Part model, mm, in its own coordinate system. Coordinates: 2 decimals unless noted, no trailing zeros. Write each loop counter-clockwise with the first axis right and the second up, starting at its lowest first coordinate (ties: lowest second). Pieces come first, ordered by that corner, then holes. Notation, with made-up numbers: (41, 80.5) -> (63, 80.5) arc R29 cw to (63, 118.5) -> close; hole circle Ø6 at (-13.75, 14.5). An arc over 180 degrees is marked (long way). Write item = value, one per line. Start each with the question number.
Q1. Band-saw the part on A-A, the plane y = 0. List the corners of the cut face in (x, z), plus the area to 3 significant figures.
Q2. Pull direction X, two halves, no side cores. Call faces 1 (the flat face through (-2, 0, 0.5)), 2 (the cylindrical face through (-1.216, 1.115, 0.303)): released by +X, released by -X, zero draft, split by the parting line, or undercut.
Q3. Pin check, flat tip, straight feed: P1, Ø1, axis at x = 0.5, y = -1, coming from the +Z side. Stop position of the tip, or through.
Q4. Probe line 1 (Y direction, x = 0, z = 0.2); line 2 (Y direction, x = 0.75, z = 0.3); line 3 (Y direction, x = 4, z = 0.15). List the from-to ranges inside material, lowest first.
from build123d import *

# Parameters (mm, degrees)
F0_R     = 7.5
F1_DEPTH = 0.5
F2_R     = 0.15
F3_R     = 1.65
F4_DEPTH = 0.4


# Not quite as in the source:
# - a feature names something its author has since deleted; it is built from what else it names


with BuildPart() as f1:
    # F0 (on Top) → F1 (new body)
    with BuildSketch(Plane.XY):
        Circle(F0_R)
    extrude(amount=F1_DEPTH)

    # F2
    f2_edges = [f1.edges().sort_by_distance(p)[0] for p in [
        (-7.5, 0, 0.5),
        (-7.5, 0, 0),
    ]]
    fillet(f2_edges, radius=F2_R)

    # F3 (on face) → F4 (cut)
    with BuildSketch(Plane.XY.offset(0.5)):
        Circle(F3_R)
    extrude(amount=-F4_DEPTH, mode=Mode.SUBTRACT)


solid = f1.part
Ans:
q1.outline = (-7.5, 0.15) arc R0.15 ccw to (-7.35, 0) -> (7.35, 0) arc R0.15 ccw to (7.5, 0.15) -> (7.5, 0.35) arc R0.15 ccw to (7.35, 0.5) -> (1.65, 0.5) -> (1.65, 0.1) -> (-1.65, 0.1) -> (-1.65, 0.5) -> (-7.35, 0.5) arc R0.15 ccw to (-7.5, 0.35) -> close
q1.area = 6.16 mm2
q2.face_1 = zero draft
q2.face_2 = undercut
q3.P1 = 0.1
q4.line_1 = -7.5 to -1.65, 1.65 to 7.5
q4.line_2 = -7.46 to -1.47, 1.47 to 7.46
q4.line_3 = -6.34 to 6.34
